The model under review builds one solid part; all positions refer to its coordinate system, in mm. Round coordinates to 2 decimals unless told otherwise and drop trailing zeros. Return JSON: item names as keys, results as strings. Group by question number.
Q1. Consider section A-A (x = 48). Count the separate pieces of the cut face and the enclosed holes in it, and give its area (3 significant figures).
Q2. To check wall thickness, follow line 1 along Y through (x, z) = (64.5, 3); line 2 along Y through (x, z) = (56, 6.25); line 3 along X through (y, z) = (-5, 7.5). State the ranges of each line that lie inside material, in increasing order.
Q3. Clearance check with flat-ended pins moving along their axes: pin 1 Ø4 at (x, z) = (94.5, 2.5) entering from +Y; pin 2 Ø4 at (x, z) = (64, 4.5) entering from -Y. State where each tip first meets the part, or that it passes through.
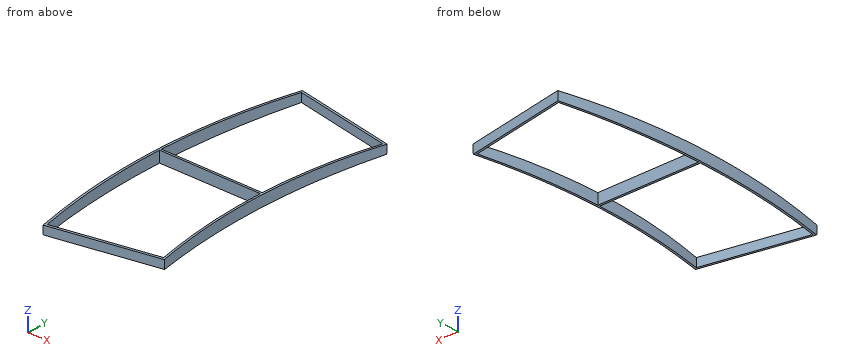
from build123d import *

# Parameters (mm, degrees)
F1_ANGLE_BACK = 11.25
F1_ANGLE      = 22.5
F2_W          = 45.7320638196
F2_H          = 22.3794019495
F2_W_2        = 176.9668050066
F2_H_2        = 15.0131394978
F2_W_3        = 53.8554313377
F4_W          = 51.5799054205
F4_H          = 20.0616745278
F5_ANGLE_BACK = 15
F5_ANGLE      = 30
F7_ANGLE_BACK = 15
F7_ANGLE      = 30
F9_DEPTH      = 25


with BuildPart() as f1:
    # F0 (on Front) → F1 (revolve)
    with BuildSketch(Plane.XZ, mode=Mode.PRIVATE) as f1_sk:
        Polygon((0.030159233, 10.9122785955), (0, 1.9123291278), (155.9991241063, 1.3895690886), (156.0292833394, 10.3895185563), align=None)
        Polygon((155.9991241063, 1.3895690886), (0, 1.9123291278), (51.0110905605, -7.2586618498), (155.9689648733, -7.610380379), align=None)
        Polygon((51.0110905605, -7.2586618498), (0, 1.9123291278), (-0.030159233, -7.0876203399), align=None)
    revolve(f1_sk.sketch.rotate(Axis((561.8991869329, 0, -48.7660320647), (-0.176947319, 0, -0.9842203241)), -F1_ANGLE_BACK), axis=Axis((561.8991869329, 0, -48.7660320647), (-0.176947319, 0, -0.9842203241)), revolution_arc=F1_ANGLE)

    # F2 (on Front) → F3 (revolve, cut)
    with BuildSketch(Plane.XZ):
        with Locations((16.1339680902, 18.1897009747)):
            Rectangle(F2_W, F2_H)
        with Locations((82.3720288345, -6.5065697489)):
            Rectangle(F2_W_2, F2_H_2)
        with Locations((143.9277156689, 18.1897009747)):
            Rectangle(F2_W_3, F2_H)
    revolve(axis=Axis((584.9095582962, 0, -6.0216095299), (0, 0, -1)), mode=Mode.SUBTRACT)

    # F4 (on Front) → F5 (revolve, cut)
    with BuildSketch(Plane.XZ, mode=Mode.PRIVATE) as f5_sk:
        Polygon((40.5, 12.6220593229), (-10.8453575522, 12.6220593229), (-10.8453575522, -3.9136288688), (17.7529230866, -3.9136288688), (40.5, -3.9136288688), align=None)
        with Locations((141.2899527103, 6.1172083952)):
            Rectangle(F4_W, F4_H)
    revolve(f5_sk.sketch.rotate(Axis((513.9181956959, 0, -119.0054643705), (0.3118081533, 0, 0.9501450813)), -F5_ANGLE_BACK), axis=Axis((513.9181956959, 0, -119.0054643705), (0.3118081533, 0, 0.9501450813)), revolution_arc=F5_ANGLE, mode=Mode.SUBTRACT)

    # F6 (on Front) → F7 (revolve, cut)
    with BuildSketch(Plane.XZ, mode=Mode.PRIVATE) as f7_sk:
        Polygon((16.4002180099, 17.1660631895), (0.0234571812, 8.9122898249), (156.0225812876, 8.3895297857), (144.173130393, 14.4683616236), align=None)
    revolve(f7_sk.sketch.rotate(Axis((561.8991869329, 0, -48.7660320647), (-0.176947319, 0, -0.9842203241)), -F7_ANGLE_BACK), axis=Axis((561.8991869329, 0, -48.7660320647), (-0.176947319, 0, -0.9842203241)), revolution_arc=F7_ANGLE, mode=Mode.SUBTRACT)

    # F8 (on face) → F9 (cut)
    with BuildSketch(Plane(origin=(0, 0, 1), x_dir=(1, 0, 0), z_dir=(0, 0, -1))):
        with BuildLine():
            Line((122.5469334165, 86.236710341), (51.8850553165, 100.0704402238))
            ThreePointArc((51.8850553165, 100.0704402238), (44.5142638986, 50.6519175795), (42.0005498992, 0.7500119204))
            Line((42.0005498992, 0.7500119204), (114.0006402026, 0.7500119204))
            ThreePointArc((114.0006402026, 0.7500119204), (116.1790999014, 43.7027715868), (122.5469334165, 86.236710341))
        make_face()
        with BuildLine():
            Line((114.0006401619, -0.7499880796), (42.0005498643, -0.7499880796))
            ThreePointArc((42.0005498643, -0.7499880796), (44.5142627181, -50.6519057176), (51.8850553165, -100.0704402238))
            Line((51.8850553165, -100.0704402238), (122.5469334165, -86.236710341))
            ThreePointArc((122.5469334165, -86.236710341), (116.1790987156, -43.7027597256), (114.0006401619, -0.7499880796))
        make_face()
    extrude(amount=-F9_DEPTH, mode=Mode.SUBTRACT)


solid = f1.part
Values:
{
 "1": {"separate pieces": "3", "enclosed holes": "0", "area": "136 mm2"},
 "2": {"line 1": "y = -99.2 to -97.6, -0.75 to 0.75, 97.6 to 99.2", "line 2": "y = -100.98 to -99.26, -0.75 to 0.75, 99.26 to 100.98", "line 3": "x = 40.52 to 42.02, 114.03 to 115.53"},
 "3": {"pin 1": "stops at y = 93.71", "pin 2": "stops at y = -99.75"}
}
